from build123d import *

# Parameters (mm, degrees)
ESQUISSE1_R                = 38.1
BOSS_EXTRU_1_DEPTH         = 51.8
ESQUISSE2_R                = 6.35
ENL_V_MAT_EXTRU_1_DEPTH    = 4.7
ESQUISSE3_R                = 5.588
ENL_V_MAT_EXTRU_2_DEPTH    = 4
ESQUISSE4_R                = 25.4
ENL_V_MAT_EXTRU_3_DEPTH    = 43.1
ESQUISSE6_OUTSIDE_W        = 102.114
ESQUISSE6_OUTSIDE_H        = 102.114
ESQUISSE6_OUTSIDE_R        = 31.75
ENL_V_MAT_EXTRU_4_DEPTH    = 2
R_P_TITION_LIN_AIRE1_COUNT = 10
R_P_TITION_LIN_AIRE1_PITCH = 4
ENL_V_START                = -2
ESQUISSE7_R                = 25.4
ENL_V_MAT_EXTRU_5_DEPTH    = 2


with BuildPart() as part:
    # Esquisse1 → Boss.-Extru.1 (new body)
    with BuildSketch(Plane.XY):
        with Locations(Location((0, 0, 0), (0, 0, 180))):
            Circle(ESQUISSE1_R)
    extrude(amount=BOSS_EXTRU_1_DEPTH)

    # Esquisse2 → Enlèv. mat.-Extru.1 (cut)
    with BuildSketch(Plane.XY.offset(51.8)):
        Circle(ESQUISSE2_R)
    extrude(amount=-ENL_V_MAT_EXTRU_1_DEPTH, mode=Mode.SUBTRACT)

    # Esquisse3 → Enlèv. mat.-Extru.2 (cut)
    with BuildSketch(Plane.XY.offset(47.1)):
        Circle(ESQUISSE3_R)
    extrude(amount=-ENL_V_MAT_EXTRU_2_DEPTH, mode=Mode.SUBTRACT)

    # Esquisse4 → Enlèv. mat.-Extru.3 (cut)
    with BuildSketch(Plane.XY.offset(43.1)):
        Circle(ESQUISSE4_R)
    extrude(amount=-ENL_V_MAT_EXTRU_3_DEPTH, mode=Mode.SUBTRACT)

    # Esquisse6 outside → Enlèv. mat.-Extru.4 (cut)
    with BuildSketch(Plane(origin=(0, 0, 0), x_dir=(-1, 0, 0), z_dir=(0, 0, -1))):
        Rectangle(ESQUISSE6_OUTSIDE_W, ESQUISSE6_OUTSIDE_H)
        Circle(ESQUISSE6_OUTSIDE_R, mode=Mode.SUBTRACT)
    enl_v_mat_extru_4 = extrude(amount=-ENL_V_MAT_EXTRU_4_DEPTH, mode=Mode.SUBTRACT)

    # Répétition linéaire1: Enlèv. mat.-Extru.4 ×10
    with Locations(*[(0, 0, i * R_P_TITION_LIN_AIRE1_PITCH) for i in range(1, R_P_TITION_LIN_AIRE1_COUNT)]):
        add(enl_v_mat_extru_4, mode=Mode.SUBTRACT)

    # Esquisse7 → Enlèv. mat.-Extru.5 (cut)
    with BuildSketch(Plane(origin=(0, 0, 43.1), x_dir=(-1, 0, 0), z_dir=(0, 0, -1)).offset(ENL_V_START)):
        with Locations(Location((0, 0, 0), (0, 0, 180))):
            Circle(ESQUISSE7_R)
    extrude(amount=ENL_V_MAT_EXTRU_5_DEPTH, mode=Mode.SUBTRACT)


solid = part.part
Build history of the part. All positions in model axes, mm. A direction names the side the tool comes from. Give positions to 0.01 mm unless a question says otherwise; leave off trailing zeros. Loops run counter-clockwise (first coordinate to the right, second up) from the corner with the lowest first, then second, coordinate; pieces in that order, holes last. Notation, with made-up numbers: (-26.5, 89) - (10.5, 89) arc R20 cw to (10.5, 124) - close; hole circle Ø1 at (5.25, 56). An arc over 180 degrees is marked (long way). Write item = value, one per line. Start each with the question number.
1) Band-saw the part on C-C on z = 33. Give the cut face in (x, y).
2) Drop flat-ended pins along their axis: pin 1 Ø10 at (x, z) = (-23.5, 36.5) entering from -Y; pin 2 Ø6 at (x, z) = (10.5, 39) entering from -Y; pin 3 Ø8 at (y, z) = (-18, 16.5) entering from -X. Give the stop position or say it passes through.
3) Tool access for faces 1 (the flat face through (9, 31, 2)), 2 (the cylindrical face through (-1.38, -6.2, 49.48)), 3 (the flat face through (9, 31, 14)): list every direction of +Z, -Z, +X, -X, +Y, -Y with a clear straight run to the whole face (end or side of a thin tool).
4) Probe probe 1 along Y at (x, z) = (0, 33); probe 2 along Y at (x, z) = (0, 46.3); probe 3 along X at (y, z) = (-14, 31.5). List the from-to ranges inside material, lowest first. Write a range as from..to.
5) Pull direction X, two halves, no side cores. Call faces 4 (the flat face through (9, 31, 6)), 5 (the cylindrical face through (-5.506, -24.796, 22.866)), 6 (the cylindrical face through (6.883, -30.995, 12.986)): +X half, -X half, draft (parallel to the pull), parting line (faces both ways), or undercut.
6) Band-saw the part on B-B on y = -33. Count the separate pieces of the cut face and the enclosed holes in it, plus the area to 3 significant figures.
7) Band-saw the part on A-A on z = 39.5. Give the cut face in (x, y), plus the area to 3 significant figures.
Final values:
q1.outline = circle Ø63.5 at (0, 0); hole circle Ø50.8 at (0, 0)
q2.pin_1 = -33.29
q2.pin_2 = -37.35
q2.pin_3 = -35.42
q3.face_1 = -Z
q3.face_2 = +Z
q3.face_3 = none
q4.probe_1 = -31.75..-25.4, 25.4..31.75
q4.probe_2 = -38.1..-5.59, 5.59..38.1
q4.probe_3 = -35.43..-21.19, 21.19..35.43
q5.face_4 = draft
q5.face_5 = undercut
q5.face_6 = parting line
q6.separate_pieces = 10
q6.enclosed_holes = 0
q6.area = 1,210 mm²
q7.outline = circle Ø76.2 at (0, 0); hole circle Ø50.8 at (0, 0)
q7.area = 2,530 mm²
